Verification items for this drawing (mm, ordinates from the low corner). Round coordinates to 2 decimals unless told otherwise and drop trailing zeros. Order: outer loops, then holes, each group sorted by start corner. A loop starts at its lowest first (then second) coordinate and runs counter-clockwise, first axis right, second up. Notation, with made-up numbers: (-33.5, 39) - (9.5, 39) arc R30 cw to (9.5, 63) - close; hole circle Ø5 at (66.5, -19). An arc over 180 degrees is marked (long way). Use a Markdown table: item, result. Add a question column.
(1) Thickness scan on line 1 along Z through (x, y) = (8, 6.25); line 2 along Y through (x, z) = (0.5, 33.5) (1 decimal); line 3 along Y through (x, z) = (1.5, 6.5) (1 decimal). Record the ranges inside material, lowest first. Write a range as [from, to].
(2) Section check B-B on y = 4.5. Record the boundary of the cut face in (x, z) (1 decimal).
(3) Gauge pin test, flat end, axial feed: P1, Ø5, axis at x = 3.5, y = 6, coming from the +Z side. Record the tip position at first contact, or that the pin passes through.
(4) Mould release check, pull along Y, two halves, no side actions. Record for the marked faces 1, 2, 3 and 4: released by +Y, released by -Y, zero draft, split by the parting line, or undercut.
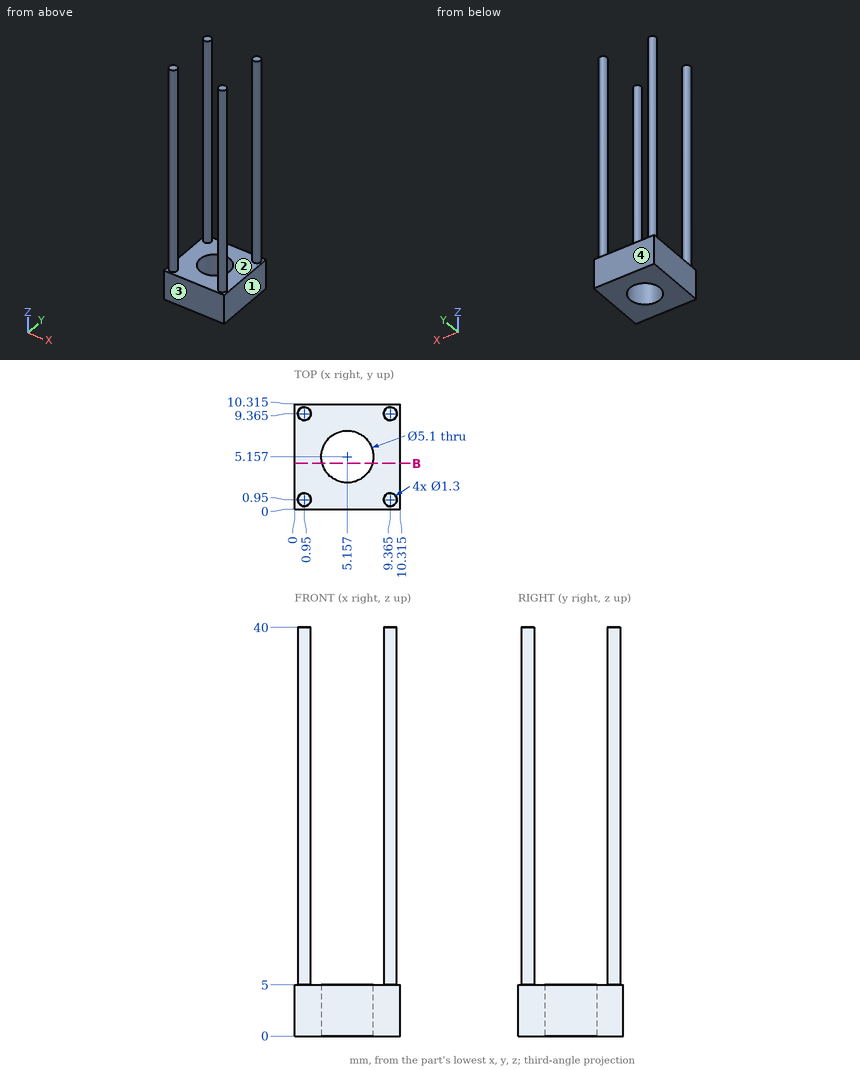
Check sheet entries:
| question | item | result |
|---|---|---|
| 1 | line 1 | z = [0, 5] |
| 1 | line 2 | y = [0.5, 1.4], [8.9, 9.8] |
| 1 | line 3 | y = [0.6, 1.3], [9, 9.7] |
| 2 | outline | (0, 0) - (2.7, 0) - (2.7, 5) - (0, 5) - close; (7.6, 0) - (10.3, 0) - (10.3, 5) - (7.6, 5) - close |
| 3 | P1 | stops at z = 5 |
| 4 | face 1 | zero draft |
| 4 | face 2 | undercut |
| 4 | face 3 | released by -Y |
| 4 | face 4 | released by +Y |
